Build history of the part. All positions in model axes, mm. A direction names the side the tool comes from. Coordinates: 2 decimals unless noted, no trailing zeros. Order: outer loops, then holes, each group sorted by start corner. A loop starts at its lowest first (then second) coordinate and runs counter-clockwise, first axis right, second up. Notation, with made-up numbers: M -28.5,-28.75 L -16.5,-28.75 A21 ccw -16.5,-10.75 Z; hole C 62.5,10.5 d2. An arc over 180 degrees is marked long. Write item = value, one per line. Start each with the question number.
Q1. Band-saw the part on D-D on y = -12.5. Write the cut outline in (x, z).
Q2. 3-axis set-ups, long thin cutter, end or side, ignore diameter. For faces 1 (the face through (0.2, -4, 53)), 2 (the face through (1.412, -0.224, 63.838)), 3 (the face through (11, -14, 27)), 4 (the face through (2.2, 0, 57)), 5 (the face through (7.2, -15, 28)): which of +Z, -Z, +X, -X, +Y, -Y reach the whole face in a straight line?
Q3. Pull direction Z, two halves, no side cores. Call faces 6 (the face through (11, 1, 52.37)), 7 (the face through (4, -15, 35.8)), 8 (the face through (25, 0, 27)): released by +Z, released by -Z, zero draft, split by the parting line, or undercut.
Q4. Pin check, flat tips, straight feed: P1, Ø12, axis at x = 15.5, y = 12, coming from the +Z side; P2, Ø3, axis at y = -1.5, z = 58, coming from the +X side; P3, Ø2, axis at y = -14.5, z = 7, coming from the -X side. Stop position of each tip, or through.
Q5. Band-saw the part on A-A on x = 3.75. Write the cut outline in (y, z).
Q6. Drill centre lines: probe 1 along X at (y, z) = (-4, 44.5); probe 2 along Z at (x, y) = (19, 5); probe 3 along Y at (x, z) = (2.25, 51.5). Where is each one in solid material? Low to high.
Q7. Band-saw the part on C-C on x = 10.5. Write the cut outline in (y, z), plus the area to 3 significant figures.
Q8. Band-saw the part on B-B on z = 35. Write the cut outline in (x, y), plus the area to 3 significant figures.
Autodesk Inventor part; units mm, degrees
ref_plane "YZ Plane" through (0, 0, 0) normal (1, 0, 0) x (0, 1, 0)
ref_plane "XZ Plane" through (0, 0, 0) normal (0, 1, 0) x (-1, 0, 0)
ref_plane "XY Plane" through (0, 0, 0) normal (0, 0, 1) x (1, 0, 0)
sketch "Sketch1" plane through (0, 0, 0) normal (0, 1, 0) x (-1, 0, 0)
  line L0 (-0.0003, 59.6701) -> (0.6603, 62.5452)
  line L1 (-2.25, 66.2) -> (-5.2, 66.2)
  line L2 (0, 19.4) -> (-7, 19.4)
  line L3 (-7, 19.4) -> (-7, 35.6)
  line L4 (-7, 35.6) -> (0, 35.6)
  arc A0 (0.6603, 62.5452) -> (-2.25, 66.2) centre (1.5, 66.2) ccw
  arc A1 (3, 59.6701) -> (-5.2, 66.2) centre (1.5, 66.2) ccw
  arc A2 (0.6603, 62.5452) -> (-2.25, 66.2) centre (1.5, 66.2) ccw
  line L5 (0, 35.6) -> (0, 59.6701)
  line L6 (1.5, 66.2) -> (-2.25, 66.2)
  line L7 (1.5, 66.2) -> (0.6603, 62.5452)
  line L8 (1.5, 66.2) -> (-5.2118, 66.0064)
  arc A3 (-2.2484, 66.0919) -> (0.5552, 62.571) centre (1.5, 66.2) ccw
  line L9 (-0.2, 52.3701) -> (-23, 52.3701)
  line L10 (-25, 54.1701) -> (-2.2, 54.1701)
  line L11 (-23, 2.2) -> (-23, 52.3701)
  line L12 (0, 0) -> (0, 19.4)
  line L13 (-24.1293, 0) -> (0, 0)
  line L14 (-25, 0) -> (-24.1293, 0)
  line L15 (-25, 0.2) -> (-0.2, 0.2)
  line L16 (-0.2, 0.2) -> (-0.2, 2.2)
  line L17 (-0.2, 2.2) -> (-23, 2.2)
  line L18 (-25, 0.2) -> (-25, 54.1701)
  line L19 (-23, 2.2) -> (-23, 0.2)
  circle A4 centre (1.5, 66.2) radius 6.7
  line L20 (-0.2, 52.3701) -> (-0.2, 59.7193)
  line L21 (0.5552, 62.571) -> (-0.2, 59.7193)
  line L22 (-2.2, 54.1701) -> (-2.2, 60.6143)
  point P0 (-5.1972, 66.0068)
  dimension "d14" = 1.652
  dimension "d18" = 22.8
  dimension "d21" = 24.8
  dimension "d22" = 0.2
  dimension "d23" = 2
extrude "Extrusion1" add sketch "Sketch1" along normal mid plane 32 contours L20 L9 L11 L19 L15 L18 L10 L22 A4 | A4 L8 A3 L21
sketch "Sketch2" plane through (0, -16, 0) normal (0, -1, 0) x (1, 0, 0)
  spline S0 degree 3 poles (24.1293, 0) (23.5574, -0.0479) (22.9856, -0.0965) (22.4138, -0.1456) (19.2606, -0.4164) (16.108, -0.6985) (8.6399, -1.2015) (4.3202, -1.3606) (0, -1.3606) (-4.3202, -1.3606) (-8.6399, -1.2015) (-16.108, -0.6985) (-19.2606, -0.4164) (-22.4138, -0.1456) (-23.2758, -0.0716) (-24.1378, 0.0014) (-25, 0.0722) knots -0.172158 -0.172158 -0.172158 -0.172158 0 0 0 0.949465 0.949465 2.245518 2.245518 2.245518 3.54157 3.54157 4.491036 4.491036 4.491036 4.750564 4.750564 4.750564 4.750564
  line L0 (24.1293, 0) -> (0, 0)
  line L1 (0, 0) -> (0, 19.4)
  line L2 (0, 19.4) -> (7, 19.4)
  line L3 (7, 35.6) -> (7, 19.4)
  line L4 (0, 35.6) -> (7, 35.6)
  line L5 (0, 35.6) -> (0, 59.6701)
  arc A0 (0, 59.6701) -> (0.0003, 59.6701) centre (-1.5, 66.2) ccw
  line L6 (0.0003, 59.6701) -> (-0.6603, 62.5452)
  arc A1 (2.25, 66.2) -> (-0.6603, 62.5452) centre (-1.5, 66.2) ccw
  line L7 (2.25, 66.2) -> (5.2, 66.2)
  arc A2 (5.2, 66.2) -> (-3, 59.6701) centre (-1.5, 66.2) ccw
  line L8 (-3, 59.6701) -> (-3, 4.75)
  line L9 (-25, 4.75) -> (-3, 4.75)
  line L10 (-25, 0.0722) -> (-25, 4.75)
  line L11 (0, 21.4) -> (6, 21.4)
  line L12 (0, 21.4) -> (0, 33.6)
  line L13 (0, 33.6) -> (6, 33.6)
  line L14 (6, 33.6) -> (6, 21.4)
  line L15 (0, 35.8) -> (7.2, 35.8)
  line L16 (7.2, 35.8) -> (7.2, 19.2)
  line L17 (7.2, 19.2) -> (0, 19.2)
  line L18 (0, 19.2) -> (0, 35.8)
  line L19 (0.2, 52.3701) -> (23, 52.3701)
  line L20 (0.2, 52.3701) -> (0.2, 35.8)
  line L21 (0.2, 19.2) -> (0.2, 0.2)
  line L22 (23, 0.2) -> (25, 0.2)
  line L23 (23, 52.3701) -> (23, 0.2)
  line L24 (0.2, 0.2) -> (23, 0.2)
  dimension "d24" = 7.2
  dimension "d25" = 16.6
  dimension "d26" = 0.2
  dimension "d27" = 0.2
extrude "Extrusion2" add sketch "Sketch2" against normal blind 2 contours L17 L16 L15 L20 L19 L23 L24 L21
equation "\"d14\" = d17"
properties part number "prototype_12_cover"
Recorded:
q1.outline = M -0.56,62.57 L 0.2,59.72 L 0.2,52.37 L 23,52.37 L 23,0.2 L 25,0.2 L 25,54.17 L 2.2,54.17 L 2.2,60.61 A6.7 ccw 5.2,66.01 L 2.25,66.09 A3.75 cw Z
q2.face_1 = -Z, -X, +Y, -Y
q2.face_2 = +Z, -X, +Y, -Y
q2.face_3 = -Z, -X, +Y
q2.face_4 = +X, +Y, -Y
q2.face_5 = -X, +Y, -Y
q3.face_6 = released by -Z
q3.face_7 = undercut
q3.face_8 = zero draft
q4.P1 = 54.17
q4.P2 = 2.2
q4.P3 = 0.2
q5.outline = M -16,0.2 L -14,0.2 L -14,19.2 L -16,19.2 Z; M -16,35.8 L -14,35.8 L -14,52.37 L 16,52.37 L 16,54.17 L -16,54.17 Z; M -16,62.04 L 16,62.04 L 16,66.05 L -16,66.05 Z
q6.probe_1 = 23 to 25
q6.probe_2 = 52.37 to 54.17
q6.probe_3 = -16 to -14
q7.outline = M -16,0.2 L -14,0.2 L -14,52.37 L 16,52.37 L 16,54.17 L -16,54.17 Z
q7.area = 162 mm2
q8.outline = M 7.2,-16 L 25,-16 L 25,16 L 23,16 L 23,-14 L 7.2,-14 Z
q8.area = 95.6 mm2
